from build123d import *

# Parameters (mm, degrees)
F0_W     = 50.8
F0_H     = 19.05
F1_DEPTH = 10
F3_DEPTH = 6
F5_DEPTH = 19.05
F7_DEPTH = 5


with BuildPart() as f1:
    # F0 (on Top) → F1 (new body)
    with BuildSketch(Plane.XY):
        Rectangle(F0_W, F0_H)
    extrude(amount=F1_DEPTH)

    # F2 (on face) → F3 (cut)
    with BuildSketch(Plane(origin=(0, 0, 0), x_dir=(1, 0, 0), z_dir=(0, 0, -1))):
        with BuildLine():
            ThreePointArc((-12.875006, 0), (-16.050006, 3.175), (-19.225006, 0))
            Line((-19.225006, 0), (-12.875006, 0))
        make_face()
        with BuildLine():
            ThreePointArc((19.225006, 0), (16.050006, 3.175), (12.875006, 0))
            Line((12.875006, 0), (19.225006, 0))
        make_face()
        with BuildLine():
            Line((19.225006, 0), (12.875006, 0))
            ThreePointArc((12.875006, 0), (16.050006, -3.175), (19.225006, 0))
        make_face()
        with BuildLine():
            Line((-12.875006, 0), (-19.225006, 0))
            ThreePointArc((-19.225006, 0), (-16.050006, -3.175), (-12.875006, 0))
        make_face()
    extrude(amount=-F3_DEPTH, mode=Mode.SUBTRACT)

    # F4 (on face) → F5 (join)
    with BuildSketch(Plane(origin=(0, 0, 0), x_dir=(1, 0, 0), z_dir=(0, 0, -1))):
        Polygon((-25.4, -4.525), (-25.4, -9.525), (-2.5, -9.525), (2.5, -9.525), (25.4, -9.525), (25.4, -4.525), (25.4, 9.525), (21.59, 9.525), (21.59, -4.525), (-2.5, -4.525), (-21.59, -4.525), (-21.59, 9.525), (-25.4, 9.525), align=None)
    extrude(amount=F5_DEPTH)

    # F6 (on face) → F7 (cut, through all)
    with BuildSketch(Plane(origin=(0, 9.525, 0), x_dir=(-1, 0, 0), z_dir=(0, 1, 0))):
        with BuildLine():
            Line((0, -9.525), (2.6, -9.525))
            ThreePointArc((2.6, -9.525), (1.838478, -7.686522), (0, -6.925))
            Line((0, -6.925), (0, -9.525))
        make_face()
        with BuildLine():
            ThreePointArc((0, -12.125), (1.838478, -11.363478), (2.6, -9.525))
            Line((2.6, -9.525), (0, -9.525))
            Line((0, -9.525), (0, -12.125))
        make_face()
        with BuildLine():
            Line((0, -9.525), (0, -6.925))
            ThreePointArc((0, -6.925), (-1.838478, -7.686522), (-2.6, -9.525))
            Line((-2.6, -9.525), (0, -9.525))
        make_face()
        with BuildLine():
            ThreePointArc((-2.6, -9.525), (-1.838478, -11.363478), (0, -12.125))
            Line((0, -12.125), (0, -9.525))
            Line((0, -9.525), (-2.6, -9.525))
        make_face()
    extrude(amount=-F7_DEPTH, mode=Mode.SUBTRACT)


solid = f1.part
Could you check a few things on this model? Use its own coordinates, in mm. A direction names the side the tool comes from. Round coordinates to 2 decimals unless told otherwise and drop trailing zeros. Order: outer loops, then holes, each group sorted by start corner. A loop starts at its lowest first (then second) coordinate and runs counter-clockwise, first axis right, second up.
Q1. Please list where these lines run through material, in increasing order: probe 1 along X at (y, z) = (-5.75, -4); probe 2 along Z at (x, y) = (-13.5, -8); probe 3 along Y at (x, z) = (5, -7.75) (3 decimals).
Geometry says:
probe 1: x = -25.4 to -21.59, 21.59 to 25.4
probe 2: z = 0 to 10
probe 3: y = 4.525 to 9.525
Q2. Which directions (+Z, -Z, +X, -X, +Y, -Y) give clear straight access to the entire face, cutting with the end or side of a thin tool? Please do faces 1 (the face through (21.59, -3, -9)), 2 (the face through (0, -9.525, 2)), 3 (the face through (16, 0, 6)).
Geometry says:
face 1: -Z, -Y
face 2: +Z, -Z, +X, -X, -Y
face 3: -Z
Q3. I'm going to push flat-ended pins straight in: P1, Ø1.9, axis at x = -15, y = -1.5, coming from the -Z side; P2, Ø9.5, axis at x = 8.5, z = -7, coming from the -Y side (3 decimals); P3, Ø11, axis at x = -1.5, y = -5, coming from the -Z side. Where does each tip first touch, or does it pass through?
Geometry says:
P1: stops at z = 6
P2: stops at y = 4.525
P3: stops at z = 0
Q4. Imagine slicing it at B-B, the plane z = -13. List the corners of the cut face in (x, y) for me (3 decimals).
Geometry says:
outline: (-25.4, -9.525) - (-21.59, -9.525) - (-21.59, 4.525) - (21.59, 4.525) - (21.59, -9.525) - (25.4, -9.525) - (25.4, 9.525) - (-25.4, 9.525) - close
Q5. Imagine slicing it at A-A, the plane y = 0. List the corners of the cut face in (x, z) for me (3 decimals).
Geometry says:
outline: (-25.4, -19.05) - (-21.59, -19.05) - (-21.59, 0) - (-19.225, 0) - (-19.225, 6) - (-12.875, 6) - (-12.875, 0) - (12.875, 0) - (12.875, 6) - (19.225, 6) - (19.225, 0) - (21.59, 0) - (21.59, -19.05) - (25.4, -19.05) - (25.4, 10) - (-25.4, 10) - close
Q6. Imagine slicing it at D-D, the plane y = -3.75. List the corners of the cut face in (x, z) for me, then the cut area to 3 significant figures.
Geometry says:
outline: (-25.4, -19.05) - (-21.59, -19.05) - (-21.59, 0) - (21.59, 0) - (21.59, -19.05) - (25.4, -19.05) - (25.4, 10) - (-25.4, 10) - close
area: 653 mm2
Q7. Thinking about a two-plate mould opening in Y: for faces 4 (the face through (0, 9.525, -4)), 5 (the face through (0, 0, 10)), 6 (the face through (13.02, 0.95, 2.96)), which applies, released by +Y, released by -Y, zero draft, split by the parting line, or undercut?
Geometry says:
face 4: released by +Y
face 5: zero draft
face 6: undercut
Q8. Imagine slicing it at C-C, the plane x = -11.5. List the corners of the cut face in (y, z) for me (3 decimals).
Geometry says:
outline: (-9.525, 0) - (4.525, 0) - (4.525, -19.05) - (9.525, -19.05) - (9.525, 10) - (-9.525, 10) - close
